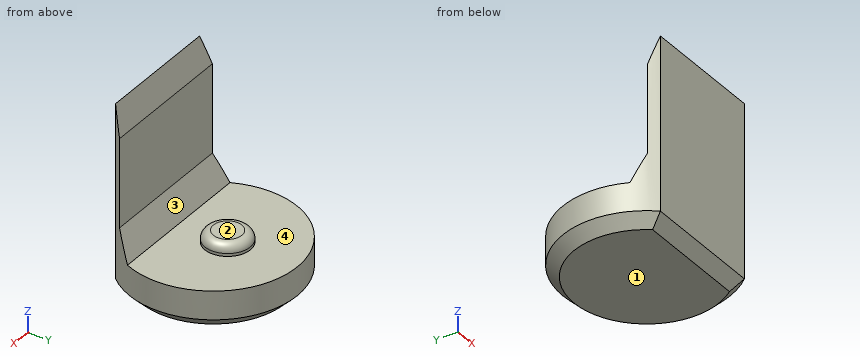
```python
from build123d import *

# Parameters (mm, degrees)
PAD008_DEPTH         = 6.5
POCKET007_DEPTH      = 2.951
POCKET007_DEPTH_BACK = 2.951
SKETCH023_R          = 0.8
PAD009_DEPTH         = 0.4
FILLET001_R          = 0.3
CHAMFER007_SIZE      = 0.4


with BuildPart() as part:
    # Sketch022 → Pad008 (new body)
    with BuildSketch(Plane.XY):
        with BuildLine():
            ThreePointArc((2.2, -1.9653244007), (0, 2.95), (-2.2, -1.9653244007))
            Line((-2.2, -1.9653244007), (2.2, -1.9653244007))
        make_face()
    extrude(amount=PAD008_DEPTH)

    # Sketch024 → Pocket007 (cut, two sides)
    with BuildSketch(Plane.YZ) as pocket007_sk:
        Polygon((-1.97, 6.5), (-1.67, 5.5), (-1.67, 2.4), (-1.22, 1.4), (4, 1.4), (4, 6.5), align=None)
    extrude(amount=-POCKET007_DEPTH, mode=Mode.SUBTRACT)
    extrude(pocket007_sk.sketch, amount=POCKET007_DEPTH_BACK, mode=Mode.SUBTRACT)

    # Sketch023 (on Face7 of Pocket007) → Pad009 (join)
    with BuildSketch(Plane.XY.offset(1.4)):
        with Locations((0, 0.5)):
            Circle(SKETCH023_R)
    extrude(amount=PAD009_DEPTH)

    # Fillet001
    fillet001_edges = [part.edges().sort_by_distance(p)[0] for p in [
        (-0.8, 0.5, 1.8),
    ]]
    fillet(fillet001_edges, radius=FILLET001_R)

    # Chamfer007
    chamfer007_edges = [part.edges().sort_by_distance(p)[0] for p in [
        (0, 2.95, 0),
        (0, -1.965324, 0),
    ]]
    chamfer(chamfer007_edges, length=CHAMFER007_SIZE)


with BuildPart() as part_1:
    # Body091 placement: moved
    add(part.part.moved(Location((0, 66, 0))))


solid = part_1.part
```
Work out the finished part from the listing and answer in its coordinate system (mm). Face numbers are marked on the shaded views. A direction names the side the tool comes from. Give positions to 0.01 mm unless a question says otherwise; leave off trailing zeros. Order: outer loops, then holes, each group sorted by start corner. A loop starts at its lowest first (then second) coordinate and runs counter-clockwise, first axis right, second up. Notation, with made-up numbers: (8.5, 87.25) - (65.5, 87.25) arc R15 cw to (65.5, 108.25) - close; hole circle Ø1 at (58, -3). An arc over 180 degrees is marked (long way). One line per item, written item: value. Start each with the question number.
1. Section C-C, the plane z = 6 is taken. Write down the section's boundary in (x, y).
2. Each of these flat-tipped pins is pushed along its axis until it touches: pin 1 Ø1.5 at (y, z) = (65, 2.5) entering from -X; pin 2 Ø0.8 at (x, y) = (0, 66.5) entering from +Z; pin 3 Ø2 at (x, y) = (2.5, 68) entering from +Z. Where does it stop, or does it pass through?
3. Which of the six approach directions +Z, -Z, +X, -X, +Y, -Y give full straight-line access (tool end or side, diameter ignored) to the marked faces 1, 2, 3 and 4?
4. Section B-B, the plane z = 4.75 is taken. Write down the section's boundary in (x, y), then the cut area to 3 significant figures.
5. Consider line 1 (Y direction, x = 0.8, z = 4); line 2 (Z direction, x = -1.2, y = 66.2); line 3 (Y direction, x = -1.85, z = 2). Determine where each line is inside the solid, lowest interval first.
6. Section A-A, the plane z = 1 is taken. Write down the section's boundary in (x, y), then the cut area to 3 significant figures.
Filled sheet:
1. outline: (-2.32, 64.18) arc R2.95 ccw to (-2.2, 64.03) - (2.2, 64.03) arc R2.95 ccw to (2.32, 64.18) - close
2. pin 1: x = -2.57
2. pin 2: z = 1.8
2. pin 3: z = 1.4
3. face 1: -Z, +X, -X, +Y, -Y
3. face 2: +Z, +X, -X, +Y
3. face 3: +Z, +X, -X
3. face 4: +Z
4. outline: (-2.43, 64.33) arc R2.95 ccw to (-2.2, 64.03) - (2.2, 64.03) arc R2.95 ccw to (2.43, 64.33) - close
4. area: 1.37 mm²
5. line 1: 64.03 to 64.33
5. line 2: 0 to 1.4
5. line 3: 64.03 to 64.51
6. outline: (-2.2, 64.03) - (2.2, 64.03) arc R2.95 ccw (long way) to start
6. area: 24.3 mm²
